Source: CAD feature listing. Evaluate the final solid. Frame: model axes, mm. A direction names the side the tool comes from. Round coordinates to 2 decimals unless told otherwise and drop trailing zeros. Order: outer loops, then holes, each group sorted by start corner. A loop starts at its lowest first (then second) coordinate and runs counter-clockwise, first axis right, second up. Notation, with made-up numbers: (-31, 7) - (-21, 7) arc R17 cw to (-21, 30) - close; hole circle Ø5 at (-39, 19). An arc over 180 degrees is marked (long way). Put each result on its own line as item: value. Start each with the question number.
1) Section C-C on y = -295.5. Output: boundary loops of the cut face in (x, z) (1 decimal).
2) Access query for faces 1 (the face through (-2, -577.85, 2)), 2 (the face through (-2, -574.675, 2)). Directions: +Z, -Z, +X, -X, +Y, -Y. A direction counts if a zero-diameter tool reaches every point of the face in a straight line with its end or side. Return the directions, or none.
3) Mould query, pull axis Z, two halves, no side actions, for faces 3 (the face through (86.196, -283.315, 135.197)), 4 (the face through (2, 3.175, 2)). Classes: +Z half, -Z half, draft (parallel to the pull), parting line (faces both ways), or undercut.
4) Contact query for flat-ended pins moving along their axis: P1, Ø1.5, axis at y = -232, z = 29.5, coming from the -X side; P2, Ø8, axis at x = -18.5, y = -485.5, coming from the +Z side; P3, Ø8, axis at y = -63, z = -125.5, coming from the -X side. Output: stop coordinate, or through.
5) Line query: probe 1 along Y at (x, z) = (62, -65) (3 decimals); probe 2 along Z at (x, y) = (0, -183); probe 3 along Z at (x, y) = (38, -204). Output: solid intervals per line, ascending. Write a range as [from, to].
```python
from build123d import *

# Parameters (mm, degrees)
F0_R     = 163.5125
F0_R_2   = 160.3375
F1_DEPTH = 574.675
F2_R     = 163.5125
F3_DEPTH = 3.175
F4_R     = 163.5125
F5_DEPTH = 3.175


with BuildPart() as f1:
    # F0 (on Front) → F1 (new body)
    with BuildSketch(Plane.XZ):
        Circle(F0_R)
        Circle(F0_R_2, mode=Mode.SUBTRACT)
    extrude(amount=F1_DEPTH)

    # F2 (on face) → F3 (join)
    with BuildSketch(Plane.XZ.offset(574.675)):
        Circle(F2_R)
    extrude(amount=F3_DEPTH)

    # F4 (on face) → F5 (join)
    with BuildSketch(Plane(origin=(0, 0, 0), x_dir=(-1, 0, 0), z_dir=(0, 1, 0))):
        Circle(F4_R)
    extrude(amount=F5_DEPTH)


solid = f1.part
```
Answer sheet:
1. outline: circle Ø327 at (0, 0); hole circle Ø320.7 at (0, 0)
2. face 1: +Z, -Z, +X, -X, -Y
2. face 2: none
3. face 3: undercut
3. face 4: draft
4. P1: x = -160.97
4. P2: z = 162.87
4. P3: x = -109.43
5. probe 1: [-577.85, -574.675], [0, 3.175]
5. probe 2: [-163.51, -160.34], [160.34, 163.51]
5. probe 3: [-159.04, -155.77], [155.77, 159.04]
